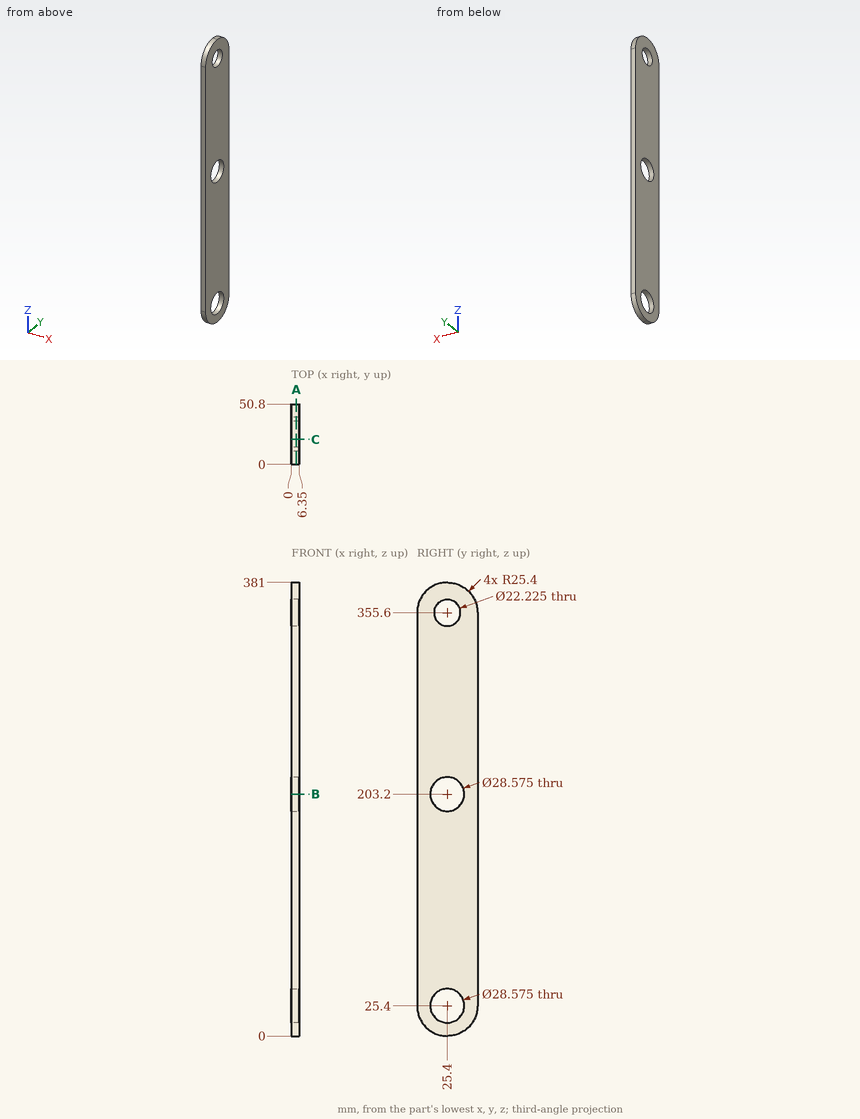
Geometry: see drawing. Coordinates: mm, zero at the bounding-box minimum. Coordinates: 2 decimals unless noted, no trailing zeros. Loops run counter-clockwise (first coordinate to the right, second up) from the corner with the lowest first, then second, coordinate; pieces in that order, holes last.
(1) Section C-C on y = 21. Return the cut outline in (x, z).
(2) Material intervals for probe 1 along Y at (x, z) = (3.5, 355.6); probe 2 along Z at (x, y) = (4, 32.5); probe 3 along Z at (x, y) = (0.75, 29), sorted ascending.
(3) Section A-A on x = 4. Count the separate pieces of the cut face and the enclosed holes in it, then the cut area to 3 significant figures.
(4) Section B-B on z = 203.2. Return the cut outline in (x, y), then the cut area to 3 significant figures.
(5) First-contact query: pin 1 Ø3 at (x, y) = (5.5, 27.5) entering from +Z; pin 2 Ø23 at (y, z) = (25.4, 25.4) entering from +X; pin 3 Ø1 at (x, y) = (1, 35) entering from -Z. Flat tips, straight axial feed; report the tip coordinate or a pass-through.
Data:
1. outline: (0, 0.38) - (6.35, 0.38) - (6.35, 11.81) - (0, 11.81) - close; (0, 38.99) - (6.35, 38.99) - (6.35, 189.61) - (0, 189.61) - close; (0, 216.79) - (6.35, 216.79) - (6.35, 345.4) - (0, 345.4) - close; (0, 365.8) - (6.35, 365.8) - (6.35, 380.62) - (0, 380.62) - close
2. probe 1: y = 0 to 14.29, 36.51 to 50.8
2. probe 2: z = 1.01 to 13, 37.8 to 190.8, 215.6 to 347.05, 364.15 to 379.99
2. probe 3: z = 0.26 to 11.57, 39.23 to 189.37, 217.03 to 345.09, 366.11 to 380.74
3. separate pieces: 1
3. enclosed holes: 3
3. area: 17,100 mm2
4. outline: (0, 0) - (6.35, 0) - (6.35, 11.11) - (0, 11.11) - close; (0, 39.69) - (6.35, 39.69) - (6.35, 50.8) - (0, 50.8) - close
4. area: 141 mm2
5. pin 1: stops at z = 380.99
5. pin 2: passes through
5. pin 3: stops at z = 1.69
